Here's how the part is built. I have some questions about the finished solid (model axes, mm). Face numbers are marked on the shaded views. Round coordinates to 2 decimals unless told otherwise and drop trailing zeros. Loops run counter-clockwise (first coordinate to the right, second up) from the corner with the lowest first, then second, coordinate; pieces in that order, holes last. Notation, with made-up numbers: (73.25, 6) - (93.25, 6) arc R24 ccw to (93.25, 17) - close; hole circle Ø10 at (28.25, -31.75). An arc over 180 degrees is marked (long way). Return JSON: item names as keys, results as strings. Group by question number.
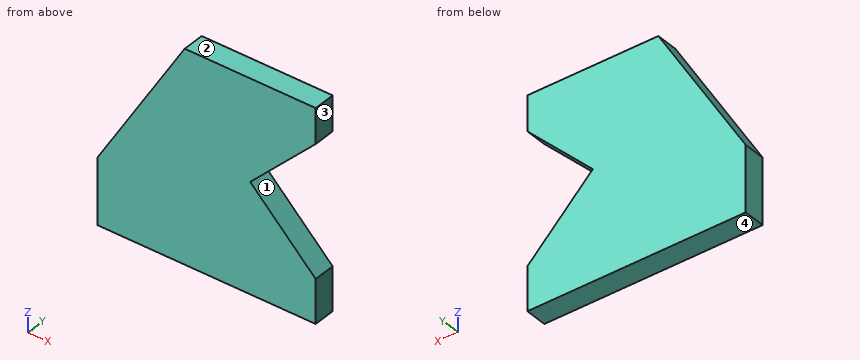
```python
from build123d import *

# Parameters (mm, degrees)
F1_DEPTH = 5


with BuildPart() as f1:
    # F0 (on Front) → F1 (new body)
    with BuildSketch(Plane.XZ):
        Polygon((0, 15), (0, 0), (35, 0), (50, 0), (50, 10), (35, 25), (50, 40), (50, 48), (20, 48), align=None)
    extrude(amount=-F1_DEPTH)


solid = f1.part
```
Q1. Imagine slicing it at D-D, the plane z = 22.5. List the corners of the cut face in (x, y) for me.
Q2. Imagine slicing it at B-B, the plane y = 3.2. List the corners of the cut face in (x, z) for me, and give its area (4 significant figures).
Q3. Imagine slicing it at C-C, the plane z = 11. List the corners of the cut face in (x, y) for me, and give its area (3 significant figures).
Q4. Imagine slicing it at A-A, the plane x = 36.5. List the corners of the cut face in (y, z) for me.
Q5. Please list where these lines run through material, in increasing order: line 1 (Z direction, x = 44.5, y = 3.55); line 2 (Z direction, x = 47.5, y = 2); line 3 (X direction, y = 3.3, z = 44.5).
Q6. If we mould it in two halves opening along Z, with no side actions, what happens to the marked faces 1, 2, 3 and 4? For each: +Z half, -Z half, draft (parallel to the pull), parting line (faces both ways), or undercut.
Q7. Will this pin go through, and if not, where does the flat tip stop? pin 1 Ø2 at (y, z) = (3.5, 9.5) entering from -X.
Output values:
{
 "1": {"outline": "(4.55, 0) - (37.5, 0) - (37.5, 5) - (4.55, 5) - close"},
 "2": {"outline": "(0, 0) - (50, 0) - (50, 10) - (35, 25) - (50, 40) - (50, 48) - (20, 48) - (0, 15) - close", "area": "1,845 mm^2"},
 "3": {"outline": "(0, 0) - (49, 0) - (49, 5) - (0, 5) - close", "area": "245 mm^2"},
 "4": {"outline": "(0, 0) - (5, 0) - (5, 23.5) - (0, 23.5) - close; (0, 26.5) - (5, 26.5) - (5, 48) - (0, 48) - close"},
 "5": {"line 1": "z = 0 to 15.5, 34.5 to 48", "line 2": "z = 0 to 12.5, 37.5 to 48", "line 3": "x = 17.88 to 50"},
 "6": {"face 1": "undercut", "face 2": "+Z half", "face 3": "draft", "face 4": "-Z half"},
 "7": {"pin 1": "stops at x = 0"}
}
